Design review of the part shown in the three views and the two pictorial views. Dimensions are in mm from the part's minimum x, y and z. A direction names the side the tool comes from. Give positions to 0.01 mm unless a question says otherwise; leave off trailing zeros. Loops run counter-clockwise (first coordinate to the right, second up) from the corner with the lowest first, then second, coordinate; pieces in that order, holes last.
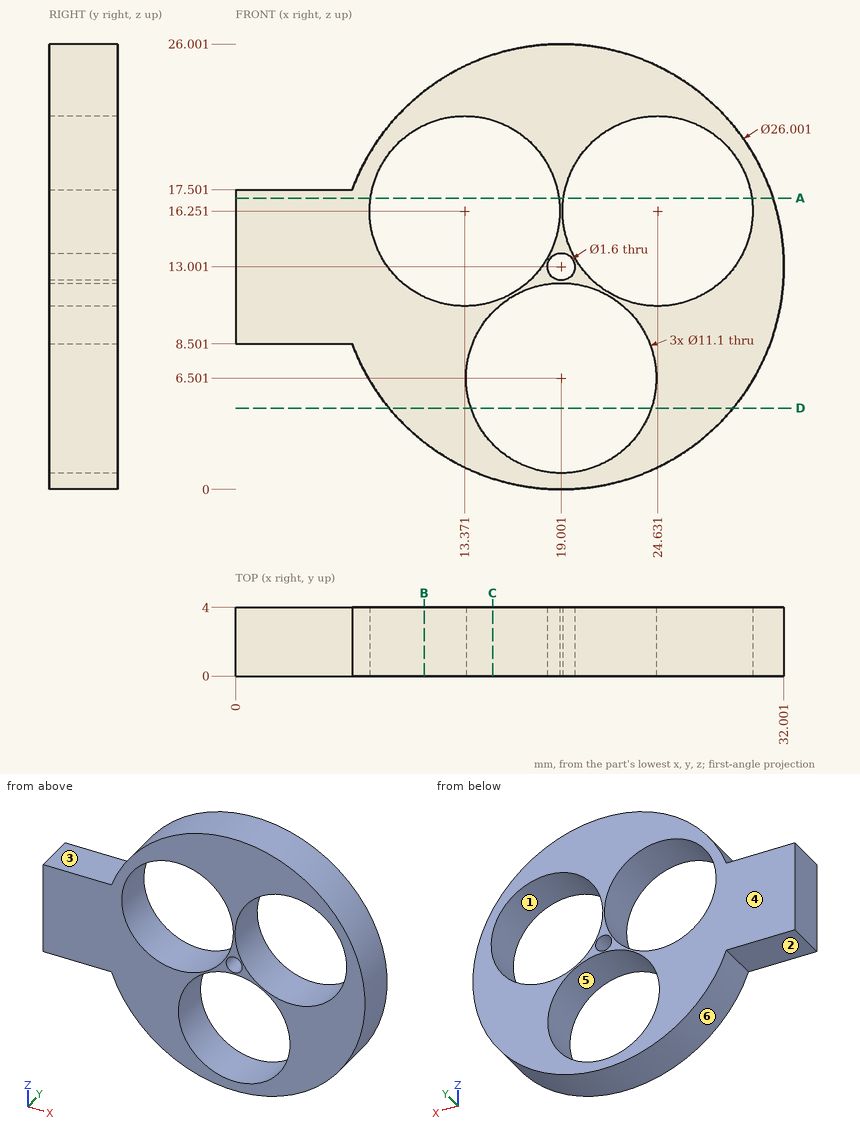
Q1. Tool access review of the marked faces 1, 2 and 3: name each direction out of +Z, -Z, +X, -X, +Y, -Y from which nothing blocks a thin tool from reaching the whole face with its end or side.
Results:
face 1: +Y, -Y
face 2: -Z, -X, +Y, -Y
face 3: +Z, -X, +Y, -Y
Q2. Wall thickness on line 1 (Z direction, x = 19.5, y = 1.45) (1 decimal); line 2 (X direction, y = 0.75, z = 18.75) (1 decimal); line 3 (Z direction, x = 14, y = 3.5) (1 decimal): over which ranges is each line inside the solid? List them lowest first.
Results:
line 1: z = 0 to 1, 12 to 12.4, 13.6 to 14.1, 18.4 to 26
line 2: x = 7.3 to 8.4, 18.3 to 19.7, 29.6 to 30.7
line 3: z = 1 to 4.1, 8.9 to 10.7, 21.8 to 25
Q3. Insertion check: pin 1 (2 mm diameter, centred on x = 17.5, z = 11.5, fed in from -Y); pin 2 (2 mm diameter, centred on y = 0.5, z = 6, fed in from +X); pin 3 (2 mm diameter, centred on x = 5, y = 3, fed in from -Z); pin 4 (10 mm diameter, centred on x = 19, z = 6.5, fed in from +Y). Each pin has a flat end and moves straight along its axis. Give the tip position at first contact, or say it passes through.
Results:
pin 1: stops at y = 0
pin 2: stops at x = 30.53
pin 3: stops at z = 8.5
pin 4: passes through
Q4. Draft analysis for pull direction X (two halves, no side actions). For the marked faces 4, 5 and 6, state which applies: pulls with the +X half, pulls with the -X half, needs draft (parallel to the pull), parting line crosses it, or undercut.
Results:
face 4: needs draft
face 5: undercut
face 6: parting line crosses it
Q5. Take a section at A-A (z = 17). Give the boundary of the cut face in (x, y).
Results:
outline: (0, 0) - (7.87, 0) - (7.87, 4) - (0, 4) - close; (18.87, 0) - (19.13, 0) - (19.13, 4) - (18.87, 4) - close; (30.13, 0) - (31.37, 0) - (31.37, 4) - (30.13, 4) - close
Q6. Take a section at B-B (x = 11). Give the boundary of the cut face in (y, z).
Results:
outline: (0, 2.75) - (4, 2.75) - (4, 11.23) - (0, 11.23) - close; (0, 21.27) - (4, 21.27) - (4, 23.25) - (0, 23.25) - close
Q7. Take a section at D-D (z = 4.75). Give the boundary of the cut face in (x, y).
Results:
outline: (8.95, 0) - (13.73, 0) - (13.73, 4) - (8.95, 4) - close; (24.27, 0) - (29.05, 0) - (29.05, 4) - (24.27, 4) - close
Q8. Take a section at C-C (x = 15). Give the boundary of the cut face in (y, z) (1 decimal).
Results:
outline: (0, 0.6) - (4, 0.6) - (4, 2.7) - (0, 2.7) - close; (0, 10.3) - (4, 10.3) - (4, 10.9) - (0, 10.9) - close; (0, 21.6) - (4, 21.6) - (4, 25.4) - (0, 25.4) - close
